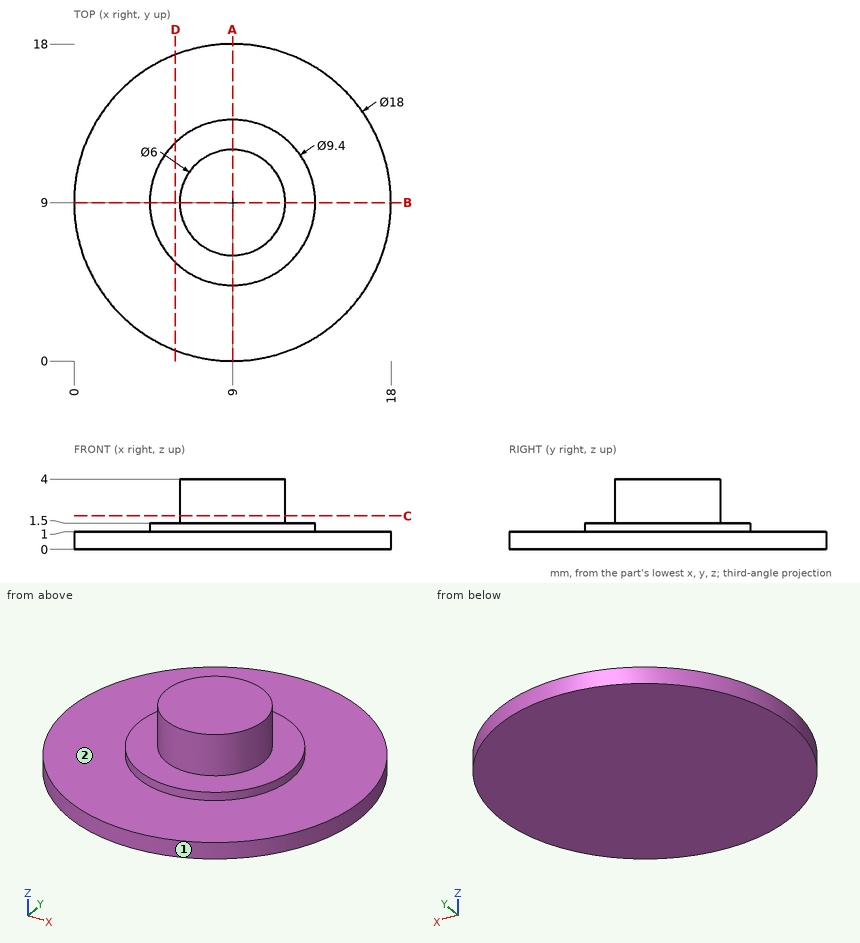
Answer from the drawing. Dimensions are ordinates in mm from the lowest x, y and z of the part. A direction names the side the tool comes from. Give positions to 0.01 mm unless a question says otherwise; leave off trailing zeros. Write each loop counter-clockwise with the first axis right and the second up, starting at its lowest first coordinate (ties: lowest second). Pieces come first, ordered by that corner, then holes. Notation, with made-up numbers: (-33, -25.5) -> (-12, -25.5) arc R18 cw to (-12, -17.5) -> close; hole circle Ø5 at (45.25, -13). An arc over 180 degrees is marked (long way). Use a Markdown table: item, result.
(1) Section D-D, the plane x = 5.75 is taken. Determine the outline of the cut face in (y, z).
Return value:
| item | result |
|---|---|
| outline | (0.61, 0) -> (17.39, 0) -> (17.39, 1) -> (12.4, 1) -> (12.4, 1.5) -> (5.6, 1.5) -> (5.6, 1) -> (0.61, 1) -> close |
(2) Flat-ended cylindrical pins translate along their axes: P1, Ø1.5, axis at y = 2, z = 1, coming from the -X side; P2, Ø1.5, axis at y = 9, z = 1, coming from the -X side; P3, Ø1.5, axis at x = 13, z = 3.5, coming from the +Y side. Find the tip coordinate at first contact, or state that the pin passes through.
Return value:
| item | result |
|---|---|
| P1 | x = 2.52 |
| P2 | x = 0 |
| P3 | through |
(3) Find the intervals of material crossed by probe 1 along Z at (x, y) = (8.75, 14.5); probe 2 along Y at (x, z) = (9.5, 2.1); probe 3 along X at (y, z) = (10.25, 1.1), in increasing order. Write a range as from..to.
Return value:
| item | result |
|---|---|
| probe 1 | 0..1 |
| probe 2 | 6.04..11.96 |
| probe 3 | 4.47..13.53 |
(4) Section C-C, the plane z = 1.9 is taken. Determine the outline of the cut face in (x, y), then the cut area to 3 significant figures.
Return value:
| item | result |
|---|---|
| outline | circle Ø6 at (9, 9) |
| area | 28.3 mm2 |
(5) For the marked faces 1 and 2, determine the directions among +Z, -Z, +X, -X, +Y, -Y from which every point of the face is accessible in a straight line to the end or side of a thin tool.
Return value:
| item | result |
|---|---|
| face 1 | +Z, -Z |
| face 2 | +Z |
(6) Section A-A, the plane x = 9 is taken. Determine the outline of the cut face in (y, z).
Return value:
| item | result |
|---|---|
| outline | (0, 0) -> (18, 0) -> (18, 1) -> (13.7, 1) -> (13.7, 1.5) -> (12, 1.5) -> (12, 4) -> (6, 4) -> (6, 1.5) -> (4.3, 1.5) -> (4.3, 1) -> (0, 1) -> close |
